The model under review builds one solid part; all positions refer to its coordinate system, in mm. Face numbers are marked on the shaded views. A direction names the side the tool comes from. Coordinates: 2 decimals unless noted, no trailing zeros. Order: outer loops, then holes, each group sorted by start corner. A loop starts at its lowest first (then second) coordinate and runs counter-clockwise, first axis right, second up. Notation, with made-up numbers: M 87.5,41.25 L 97.5,41.25 A26 ccw 97.5,65.25 Z; hole C -30.75,82.5 d8. An arc over 180 degrees is marked long. Answer in a Markdown table with one row per item.
Autodesk Inventor part; units mm, degrees
ref_plane "YZ Plane" through (0, 0, 0) normal (1, 0, 0) x (0, 1, 0)
ref_plane "XZ Plane" through (0, 0, 0) normal (0, 1, 0) x (-1, 0, 0)
ref_plane "XY Plane" through (0, 0, 0) normal (0, 0, 1) x (1, 0, 0)
sketch "Sketch1" plane through (0, 0, 0) normal (0, 0, 1) x (1, 0, 0)
  line L0 (0, 0) -> (3, 0)
  line L1 (3, 0) -> (3, 72)
  line L2 (3, 72) -> (39.1537, 72)
  line L3 (42.1537, 75) -> (0, 75)
  line L4 (0, 75) -> (0, 0)
  line L5 (42.1537, 75) -> (42.1537, 0)
  line L6 (42.1537, 0) -> (39.1537, 0)
  line L7 (39.1537, 0) -> (39.1537, 72)
  dimension "d0" = 75
  dimension "d1" = 3
  dimension "d3" = 3
extrude "Extrusion1" add sketch "Sketch1" along normal blind 40
fillet "Fillet1" radius 20 2 edges at (40.6537, 0, 40) (40.6537, 0, 0)
fillet "Fillet2" radius 20 2 edges at (1.5, 0, 40) (1.5, 0, 0)
sketch "Sketch2" plane through (42.1537, 75, 40) normal (1, 0, 0) x (0, 0, -1)
  circle A0 centre (19.8608, -53.2379) radius 5
  point P0 (40, -75)
  dimension "d8" = 10
extrude "Extrusion2" cut sketch "Sketch2" against normal blind 50
sketch "Sketch3" plane through (0, 75, 0) normal (0, 1, 0) x (1, 0, 0)
  circle A0 centre (20, -20.0234) radius 10
  line L0 (0, 0) -> (0, -40)
  dimension "d11" = 20
  dimension "d12" = 20
sketch "Sketch4" plane through (0, 75, 0) normal (0, 1, 0) x (1, 0, 0)
  point P0 (0, 0)
extrude "Extrusion3" cut sketch "Sketch3" against normal through all
fillet "Fillet3" radius 2 2 edges at (42.1537, 75, 20) (0, 75, 20)
sketch "Sketch5" plane through (2, 75, 0) normal (0, 1, 0) x (1, 0, 0)
  point P0 (-2, 0)
sketch "Sketch6" plane through (42.1537, 20, 20) normal (1, 0, 0) x (0, 0, -1)
  point P0 (20, -20)
properties part number "peca1" material "Steel, Carbon"
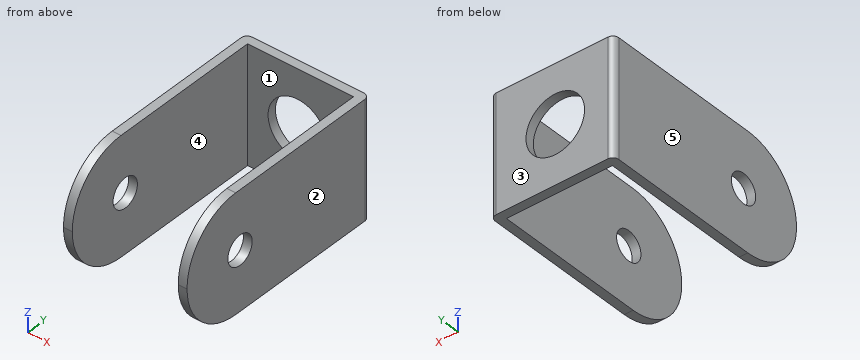
(1) Machinability: for the marked faces 4 and 5, which of the approach directions +Z, -Z, +X, -X, +Y, -Y give a long, thin tool a straight path to every point of the face, cutting with its end or side? Answer none if there is none.
Report:
| item | result |
|---|---|
| face 4 | +Z, -Z, -Y |
| face 5 | +Z, -Z, -X, +Y, -Y |
(2) Insertion check: P1, Ø8, axis at y = 22.5, z = 13.5, coming from the -X side; P2, Ø23, axis at x = 20, z = 20.02, coming from the -Y side. Each pin has a flat end and moves straight along its axis. Give the tip position at first contact, or say it passes through.
Report:
| item | result |
|---|---|
| P1 | x = 0 |
| P2 | y = 72 |
(3) Take a section at C-C (z = 28.5). Write out the cut boundary in (x, y), then the cut area to 3 significant figures.
Report:
| item | result |
|---|---|
| outline | M 0,1.9 L 3,1.9 L 3,72 L 14.69,72 L 14.69,75 L 2,75 A2 ccw 0,73 Z; M 25.31,72 L 39.15,72 L 39.15,1.9 L 42.15,1.9 L 42.15,73 A2 ccw 40.15,75 L 25.31,75 Z |
| area | 514 mm^2 |
(4) Take a section at D-D (y = 18.5). Write out the cut boundary in (x, z).
Report:
| item | result |
|---|---|
| outline | M 0,0.06 L 3,0.06 L 3,16.35 L 0,16.35 Z; M 0,23.93 L 3,23.93 L 3,39.94 L 0,39.94 Z; M 39.15,0.06 L 42.15,0.06 L 42.15,16.35 L 39.15,16.35 Z; M 39.15,23.93 L 42.15,23.93 L 42.15,39.94 L 39.15,39.94 Z |
(5) To check wall thickness, follow line 1 (X direction, y = 24.5, z = 25.5); line 2 (Z direction, x = 20, y = 74); line 3 (Y direction, x = 36.5, z = 16). State the ranges of each line that lie inside material, in increasing order. Write a range as [from, to].
Report:
| item | result |
|---|---|
| line 1 | [0, 3], [39.15, 42.15] |
| line 2 | [0, 10.02], [30.02, 40] |
| line 3 | [72, 75] |
(6) Take a section at A-A (y = 33). Write out the cut boundary in (x, z).
Report:
| item | result |
|---|---|
| outline | M 0,0 L 3,0 L 3,40 L 0,40 Z; M 39.15,0 L 42.15,0 L 42.15,40 L 39.15,40 Z |
(7) Take a section at B-B (x = 17). Write out the cut boundary in (y, z), then the cut area to 3 significant figures.
Report:
| item | result |
|---|---|
| outline | M 72,0 L 75,0 L 75,10.48 L 72,10.48 Z; M 72,29.56 L 75,29.56 L 75,40 L 72,40 Z |
| area | 62.8 mm^2 |
(8) The part is to be moulded in two halves that separate along X. For the marked faces 1, 2 and 3, say which applies: +X half, -X half, draft (parallel to the pull), parting line (faces both ways), or undercut.
Report:
| item | result |
|---|---|
| face 1 | undercut |
| face 2 | +X half |
| face 3 | draft |
